Geometry: final body of the model. Coordinates: model frame, mm. A direction names the side the tool comes from. Give positions to 0.01 mm unless a question says otherwise; leave off trailing zeros. Write each loop counter-clockwise with the first axis right and the second up, starting at its lowest first coordinate (ties: lowest second). Pieces come first, ordered by that corner, then holes. Notation, with made-up numbers: (15, 77.5) - (33, 77.5) arc R16 ccw to (33, 96.5) - close; hole circle Ø4 at (0, 20.5). An arc over 180 degrees is marked (long way). Return JSON: item names as keys, results as strings.
Autodesk Inventor part; units mm, degrees
ref_plane "Work Plane1" through (29, 0, 0) normal (-1, 0, 0) x (0, 0, 1)
ref_plane "YZ Plane" through (0, 0, 0) normal (1, 0, 0) x (0, 1, 0)
ref_plane "XZ Plane" through (0, 0, 0) normal (0, 1, 0) x (-1, 0, 0)
sketch "Sketch1" plane through (0, 0, 0) normal (0, 0, 1) x (1, 0, 0)
  line L0 (0, 0) -> (58, 0)
  line L1 (58, 0) -> (58, 28)
  line L2 (58, 28) -> (0, 28)
  line L3 (0, 28) -> (0, 0)
  dimension "d0" = 58
  dimension "d1" = 28
extrude "Extrusion1" add sketch "Sketch1" along normal blind 50
sketch "Sketch2" plane through (58, 0, 0) normal (1, 0, 0) x (0, 0, -1)
  line L0 (0, 28) -> (-50, 28)
  line L1 (0, 0) -> (-50, 0)
  line L2 (-50, 28) -> (-45, 28)
  line L3 (-45, 28) -> (-45, 0)
  line L4 (-45, 28) -> (-41, 28)
  line L5 (-41, 28) -> (-41, 0)
  line L6 (-41, 0) -> (-45, 0)
  line L7 (-45, 0) -> (-45, 28)
  dimension "d4" = 5
  dimension "d5" = 4
extrude "Extrusion2" add sketch "Sketch2" along normal blind 9
ref_plane "Work Plane1" through (29, 0, 0) normal (-1, 0, 0) x (0, 0, 1)
mirror "Mirror1" about plane through (29, 0, 0) normal (-1, 0, 0) of "Extrusion2"
sketch "Sketch3" plane through (-9, 28, 45) normal (0, 0, 1) x (1, 0, 0)
  line L0 (9, 0) -> (0, 0)
  line L1 (4.5, 0) -> (4.5, -6)
  line L2 (9, -28) -> (0, -28)
  line L3 (4.5, -6) -> (4.5, -22)
  circle A0 centre (4.5, -6) radius 2
  circle A1 centre (4.5, -22) radius 2
  dimension "d8" = 6
  dimension "d9" = 16
  dimension "d10" = 4
  dimension "d11" = 4
extrude "Extrusion3" cut sketch "Sketch3" against normal blind 9
sketch "Sketch4" plane through (58, 0, 45) normal (0, 0, 1) x (1, 0, 0)
  circle A0 centre (-62.5, 22) radius 2
  line L0 (-62.5, 22) -> (4.5, 22)
  line L1 (4.5, 22) -> (4.5, 6)
  circle A1 centre (4.5, 22) radius 2
  circle A2 centre (4.5, 6) radius 2
  point P0 (-58, 0)
  dimension "d14" = 16
  dimension "d15" = 4
  dimension "d16" = 4
extrude "Extrusion4" cut sketch "Sketch4" against normal blind 9 contours A2 | A1 L1 L0 | L0 L1 A1
sketch "Sketch5" plane through (0, 0, 50) normal (0, 0, 1) x (1, 0, 0)
  line L0 (0, 28) -> (0, 0)
  line L1 (0, 14) -> (12, 14)
  circle A0 centre (12, 14) radius 4
  dimension "d19" = 12
  dimension "d20" = 8
extrude "Extrusion5" add sketch "Sketch5" along normal blind 7
sketch "Sketch6" plane through (0, 0, 0) normal (0, 0, -1) x (-1, 0, 0)
  line L0 (0, 0) -> (-58, 0)
  line L1 (0, 28) -> (0, 0)
  line L2 (-58, 28) -> (0, 28)
  line L3 (-58, 0) -> (-58, 28)
extrude "Extrusion6" cut sketch "Sketch6" against normal blind 3
properties part number "Shoulder Servo"
Q1. Mould query, pull axis X, two halves, no side actions, for faces 1 (the cylindrical face through (60.502, 22.088, 43.028)), 2 (the cylindrical face through (8, 14, 53)), 3 (the flat face through (0, 14, 22)). Classes: pulls with the +X half, pulls with the -X half, needs draft (parallel to the pull), parting line crosses it, or undercut.
Answer key:
{"face 1": "undercut", "face 2": "parting line crosses it", "face 3": "pulls with the -X half"}
Q2. Set-up query: faces 4 (the flat face through (58, 14, 22)), 5 (the flat face through (-4, 14, 41)), 6 (the flat face through (58, 14, 47)). Return all of +Z, -Z, +X, -X, +Y, -Y with unobstructed straight access to the full face (end or side cutting, diameter ignored); none if empty.
Answer key:
{"face 4": "-Z, +X, +Y, -Y", "face 5": "-Z, -X, +Y, -Y", "face 6": "+Z, +X, +Y, -Y"}
Q3. Section query D-D, the plane y = 12.25. Return the cut outline in (x, z).
Answer key:
{"outline": "(-9, 41) - (0, 41) - (0, 3) - (58, 3) - (58, 41) - (67, 41) - (67, 45) - (58, 45) - (58, 50) - (15.6, 50) - (15.6, 57) - (8.4, 57) - (8.4, 50) - (0, 50) - (0, 45) - (-9, 45) - close"}
Q4. Material intervals for probe 1 along X at (y, z) = (22, 42.4); probe 2 along Y at (x, z) = (-4, 43); probe 3 along Z at (x, y) = (16.5, 8), sorted ascending. Write a range as [from, to].
Answer key:
{"probe 1": "x = [-9, -6.5], [-2.5, 60.5], [64.5, 67]", "probe 2": "y = [0, 4.06], [7.94, 20.06], [23.94, 28]", "probe 3": "z = [3, 50]"}
Q5. Section query B-B, the plane x = -4.5. Return the cut outline in (y, z), plus the area to 3 significant figures.
Answer key:
{"outline": "(0, 41) - (4, 41) - (4, 45) - (0, 45) - close; (8, 41) - (20, 41) - (20, 45) - (8, 45) - close; (24, 41) - (28, 41) - (28, 45) - (24, 45) - close", "area": "80.0 mm^2"}
Q6. Section query C-C, the plane x = 12. Return the cut outline in (y, z).
Answer key:
{"outline": "(0, 3) - (28, 3) - (28, 50) - (18, 50) - (18, 57) - (10, 57) - (10, 50) - (0, 50) - close"}
Q7. Section query A-A, the plane y = 6. Return the cut outline in (x, z).
Answer key:
{"outline": "(-9, 41) - (-6.5, 41) - (-6.5, 45) - (-9, 45) - close; (-2.5, 41) - (0, 41) - (0, 3) - (58, 3) - (58, 41) - (60.5, 41) - (60.5, 45) - (58, 45) - (58, 50) - (0, 50) - (0, 45) - (-2.5, 45) - close; (64.5, 41) - (67, 41) - (67, 45) - (64.5, 45) - close"}
Q8. Pin query (flat end, axial travel): P1, Ø7, axis at x = 63, y = 18.5, coming from the +Z side; P2, Ø2.5, axis at x = -4.5, y = 22, coming from the +Z side; P3, Ø14, axis at y = 13.5, z = 20, coming from the -X side; P4, Ø10, axis at x = 62.5, y = 8.5, coming from the -Z side. Return the tip coordinate at first contact, or that it passes through.
Answer key:
{"P1": "stops at z = 45", "P2": "passes through", "P3": "stops at x = 0", "P4": "stops at z = 3"}
